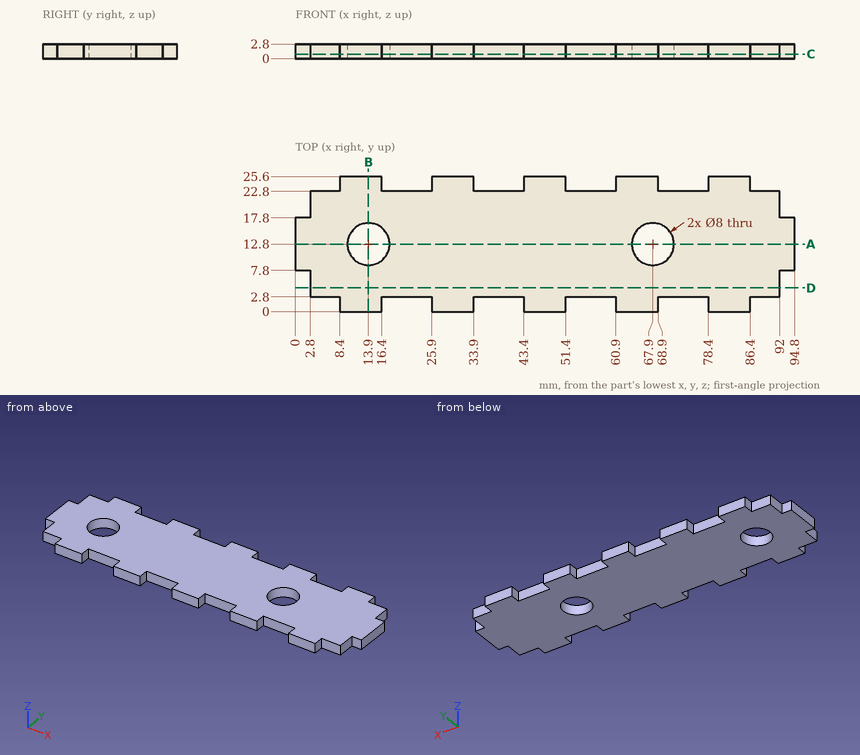
Source: three-view drawing plus pictorial views. Frame: mm from the lowest corner of the part. Round coordinates to 2 decimals unless told otherwise and drop trailing zeros. Order: outer loops, then holes, each group sorted by start corner. A loop starts at its lowest first (then second) coordinate and runs counter-clockwise, first axis right, second up. Notation, with made-up numbers: (-38, 6) -> (-27, 6) arc R22 cw to (-27, 44) -> close; hole circle Ø6 at (53, 57). An arc over 180 degrees is marked (long way). Use one line per item in the form item = value.
(1) Section A-A on y = 12.8. Return loops of the section in (x, z), and give its area (3 significant figures).
Results list:
outline = (0, 0) -> (9.9, 0) -> (9.9, 2.8) -> (0, 2.8) -> close; (17.9, 0) -> (63.9, 0) -> (63.9, 2.8) -> (17.9, 2.8) -> close; (71.9, 0) -> (94.8, 0) -> (94.8, 2.8) -> (71.9, 2.8) -> close
area = 221 mm^2
(2) First-contact query: pin 1 Ø1.4 at (y, z) = (24.5, 1) entering from -X; pin 2 Ø13 at (x, y) = (13.9, 12.8) entering from -Z; pin 3 Ø1.4 at (y, z) = (1, 0.5) entering from +X; pin 4 Ø1.4 at (x, z) = (93, 2) entering from -Y. Flat tips, straight axial feed; report the tip coordinate or a pass-through.
Results list:
pin_1 = 8.4
pin_2 = 0
pin_3 = 86.4
pin_4 = 7.8
(3) Section D-D on y = 4.5. Return loops of the section in (x, z), and give its area (3 significant figures).
Results list:
outline = (2.8, 0) -> (92, 0) -> (92, 2.8) -> (2.8, 2.8) -> close
area = 250 mm^2
(4) Section C-C on z = 0.9. Count the separate pieces of the cut face and the enclosed holes in it, and give its area (3 significant figures).
Results list:
separate_pieces = 1
enclosed_holes = 2
area = 1,960 mm^2
(5) Section B-B on x = 13.9. Return loops of the section in (y, z).
Results list:
outline = (0, 0) -> (8.8, 0) -> (8.8, 2.8) -> (0, 2.8) -> close; (16.8, 0) -> (25.6, 0) -> (25.6, 2.8) -> (16.8, 2.8) -> close
(6) Ray query, probe 1 along X at (y, z) = (12.75, 1.5); probe 2 along X at (y, z) = (23.75, 0.85); probe 3 along Y at (x, z) = (67.9, 1.4). Return the intervals inside material, ascending. Write a range as [from, to].
Results list:
probe_1 = [0, 9.9], [17.9, 63.9], [71.9, 94.8]
probe_2 = [8.4, 16.4], [25.9, 33.9], [43.4, 51.4], [60.9, 68.9], [78.4, 86.4]
probe_3 = [0, 8.8], [16.8, 25.6]
